```python
from build123d import *
from build123d.topology import SkipClean

# Parameters (mm, degrees)
SKETCH_1_R                   = 18
SKETCH_1_R_2                 = 1.3
SKETCH_1_R_3                 = 1.6
EXTRUDE_1_DEPTH              = 8
SKETCH_5_R                   = 2.1
CUT_EXTRUDE_1_DEPTH          = 6.6
HOLE_WIZARD_M3_2_D           = 3.6
HOLE_WIZARD_M3_2_CSINK_D     = 6.3
HOLE_WIZARD_M3_2_CSINK_ANGLE = 90
EXTRUDE_START                = 2
SKETCH_8_R                   = 10
SKETCH_8_R_2                 = 1.3
EXTRUDE_2_DEPTH              = 2
SKETCH_9_R                   = 10
SKETCH_9_R_2                 = 2.1
EXTRUDE_3_DEPTH              = 18
EXTRUDE_START_2              = -3.4
SKETCH_10_R                  = 2.1
SKETCH_10_R_2                = 1.25
EXTRUDE_4_DEPTH              = 3.4
SKETCH_11_R                  = 2.1
CUT_EXTRUDE_2_DEPTH          = 3.4


with BuildPart() as part:
    # 스케치1 → 보스-돌출1 (new body)
    with BuildSketch(Plane.XY):
        Circle(SKETCH_1_R)
        with Locations((0, 5.95)):
            Circle(SKETCH_1_R_2, mode=Mode.SUBTRACT)
        with Locations((5.95, 0)):
            Circle(SKETCH_1_R_2, mode=Mode.SUBTRACT)
        with Locations((0, -5.95)):
            Circle(SKETCH_1_R_2, mode=Mode.SUBTRACT)
        with Locations((-5.95, 0)):
            Circle(SKETCH_1_R_2, mode=Mode.SUBTRACT)
        with Locations((-13.249665953, 4.822484021)):
            Circle(SKETCH_1_R_3, mode=Mode.SUBTRACT)
        with Locations(Location((-13.249665953, -4.822484021, 0), (0, 0, 180))):
            Circle(SKETCH_1_R_3, mode=Mode.SUBTRACT)
        with Locations((10.801226648, 9.063305297)):
            Circle(SKETCH_1_R_3, mode=Mode.SUBTRACT)
        with Locations(Location((2.448439305, 13.885789317, 0), (0, 0, 180))):
            Circle(SKETCH_1_R_3, mode=Mode.SUBTRACT)
        with Locations((2.448439305, -13.885789317)):
            Circle(SKETCH_1_R_3, mode=Mode.SUBTRACT)
        with Locations(Location((10.801226648, -9.063305297, 0), (0, 0, 180))):
            Circle(SKETCH_1_R_3, mode=Mode.SUBTRACT)
    extrude(amount=EXTRUDE_1_DEPTH)

    # 스케치5 → 컷-돌출1 (cut)
    with BuildSketch(Plane.XY.offset(8)):
        with Locations((0, 5.95)):
            Circle(SKETCH_5_R)
        with Locations((0, -5.95)):
            Circle(SKETCH_5_R)
        with Locations((5.95, 0)):
            Circle(SKETCH_5_R)
        with Locations((-5.95, 0)):
            Circle(SKETCH_5_R)
    extrude(amount=-CUT_EXTRUDE_1_DEPTH, mode=Mode.SUBTRACT)

    # M3 접시 머리 나사용 카운터싱크2 (through all)
    with Locations(Plane(origin=(0, 0, 0), x_dir=(-1, 0, 0), z_dir=(0, 0, -1))):
        with Locations((-2.448439305, 13.885789317), (13.249665953, 4.822484021), (13.249665953, -4.822484021), (-2.448439305, -13.885789317), (-10.801226648, -9.063305297), (-10.801226648, 9.063305297)):
            CounterSinkHole(HOLE_WIZARD_M3_2_D / 2, HOLE_WIZARD_M3_2_CSINK_D / 2, counter_sink_angle=HOLE_WIZARD_M3_2_CSINK_ANGLE)

    # 스케치8 → 보스-돌출2 (add)
    with BuildSketch(Plane(origin=(0, 0, 0), x_dir=(-1, 0, 0), z_dir=(0, 0, -1)).offset(EXTRUDE_START)):
        with Locations(Location((0, 0, 0), (0, 0, 180))):
            Circle(SKETCH_8_R)
        with Locations((0, 5.95)):
            Circle(SKETCH_8_R_2, mode=Mode.SUBTRACT)
        with Locations((5.95, 0)):
            Circle(SKETCH_8_R_2, mode=Mode.SUBTRACT)
        with Locations((0, -5.95)):
            Circle(SKETCH_8_R_2, mode=Mode.SUBTRACT)
        with Locations((-5.95, 0)):
            Circle(SKETCH_8_R_2, mode=Mode.SUBTRACT)
    extrude(amount=-EXTRUDE_2_DEPTH)

    # 스케치9 → 보스-돌출3 (add)
    with SkipClean():  # the faces are left unmerged after this step: merging them gives an invalid solid
        with BuildSketch(Plane(origin=(0, 0, -2), x_dir=(-1, 0, 0), z_dir=(0, 0, -1))):
            with Locations(Location((0, 0, 0), (0, 0, 180))):
                Circle(SKETCH_9_R)
            with Locations(Location((5.95, 0, 0), (0, 0, 180))):
                Circle(SKETCH_9_R_2, mode=Mode.SUBTRACT)
            with Locations(Location((0, 5.95, 0), (0, 0, 180))):
                Circle(SKETCH_9_R_2, mode=Mode.SUBTRACT)
            with Locations(Location((-5.95, 0, 0), (0, 0, 180))):
                Circle(SKETCH_9_R_2, mode=Mode.SUBTRACT)
            with Locations(Location((0, -5.95, 0), (0, 0, 180))):
                Circle(SKETCH_9_R_2, mode=Mode.SUBTRACT)
        extrude(amount=EXTRUDE_3_DEPTH)

    # 스케치10 → 보스-돌출4 (add)
    # profile 1 of 4: a face of its own
    with SkipClean():  # the faces are left unmerged after this step: merging them gives an invalid solid
        with BuildSketch(Plane(origin=(0, 0, -20), x_dir=(-1, 0, 0), z_dir=(0, 0, -1)).offset(EXTRUDE_START_2)):
            with Locations((5.95, 0)):
                Circle(SKETCH_10_R)
            with Locations((5.95, 0)):
                Circle(SKETCH_10_R_2, mode=Mode.SUBTRACT)
        # profile 2 of 4: a face of its own
        with BuildSketch(Plane(origin=(0, 0, -20), x_dir=(-1, 0, 0), z_dir=(0, 0, -1)).offset(EXTRUDE_START_2)):
            with Locations((0, -5.95)):
                Circle(SKETCH_10_R)
            with Locations((0, -5.95)):
                Circle(SKETCH_10_R_2, mode=Mode.SUBTRACT)
        # profile 3 of 4: a face of its own
        with BuildSketch(Plane(origin=(0, 0, -20), x_dir=(-1, 0, 0), z_dir=(0, 0, -1)).offset(EXTRUDE_START_2)):
            with Locations((-5.95, 0)):
                Circle(SKETCH_10_R)
            with Locations((-5.95, 0)):
                Circle(SKETCH_10_R_2, mode=Mode.SUBTRACT)
        # profile 4 of 4: a face of its own
        with BuildSketch(Plane(origin=(0, 0, -20), x_dir=(-1, 0, 0), z_dir=(0, 0, -1)).offset(EXTRUDE_START_2)):
            with Locations((0, 5.95)):
                Circle(SKETCH_10_R)
            with Locations((0, 5.95)):
                Circle(SKETCH_10_R_2, mode=Mode.SUBTRACT)
        extrude(amount=EXTRUDE_4_DEPTH)

    # 스케치11 → 컷-돌출2 (cut)
    with BuildSketch(Plane.XY.offset(1.4)):
        with Locations((5.95, 0)):
            Circle(SKETCH_11_R)
        with Locations((0, -5.95)):
            Circle(SKETCH_11_R)
        with Locations((0, 5.95)):
            Circle(SKETCH_11_R)
        with Locations((-5.95, 0)):
            Circle(SKETCH_11_R)
    extrude(amount=-CUT_EXTRUDE_2_DEPTH, mode=Mode.SUBTRACT)


solid = part.part
```
Build history of the part. All positions in model axes, mm. A direction names the side the tool comes from. Coordinates: 2 decimals unless noted, no trailing zeros. Order: outer loops, then holes, each group sorted by start corner. A loop starts at its lowest first (then second) coordinate and runs counter-clockwise, first axis right, second up. Notation, with made-up numbers: (57.25, -32) -> (84.25, -32) arc R24 ccw to (84.25, -17) -> close; hole circle Ø3 at (37.25, 80). An arc over 180 degrees is marked (long way). Answer in a Markdown table with one row per item. Add a question column.
Q1. Band-saw the part on D-D, the plane z = -4.5. List the corners of the cut face in (x, y).
Q2. Band-saw the part on C-C, the plane x = -5.95. List the corners of the cut face in (y, z), then the cut area to 3 significant figures.
Q3. Wall check: line 1 along Y through (x, z) = (0, -10.75); line 2 along Y through (x, z) = (0, -18.9); line 3 along Z through (x, y) = (16, 0). Give the ranges that are in metal, low to high. Write a range as [from, to].
Q4. Band-saw the part on A-A, the plane y = 0. List the corners of the cut face in (x, z).
Q5. Drop flat-ended pins along their axis: pin 1 (1 mm diameter, centred on y = -8, z = -2, fed in from +X); pin 2 (1 mm diameter, centred on x = 0, y = -6.5, fed in from +Z); pin 3 (2 mm diameter, centred on x = 5.5, y = -0.5, fed in from +Z); pin 4 (12 mm diameter, centred on x = 11.5, z = -6.5, fed in from +Y). Give the stop position or say it passes through.
Q6. Band-saw the part on B-B, the plane z = 5.5. Give the number of separate pieces and of enclosed holes in the cut face, then the cut area to 3 significant figures.
Q7. Mould opens along X. For faces 1 (the face through (-2.343, 17.847, 3.944)), 2 (the face through (-1, -7, -16.6)), 3 (the face through (0, 0, -20)) say: +X half, -X half, draft (parallel to the pull), parting line (faces both ways), or undercut.
Q8. Which spindle directions (+Z, -Z, +X, -X, +Y, -Y) get a long thin tool onto all of the face, cutting with end or side? Do faces 4 (the face through (-11.6, 4.1, 4.7)), 5 (the face through (-7, -1, -16.6)). Say none if no direction does.
Answers follow:
| question | item | result |
|---|---|---|
| 1 | outline | circle Ø20 at (0, 0); hole circle Ø4.2 at (-5.95, 0); hole circle Ø4.2 at (0, -5.95); hole circle Ø4.2 at (0, 5.95); hole circle Ø4.2 at (5.95, 0) |
| 2 | outline | (-16.99, 0) -> (-8.04, 0) -> (-8.04, -20) -> (-1.25, -20) -> (-1.25, -16.6) -> (-2.1, -16.6) -> (-2.1, 8) -> (-16.99, 8) -> close; (1.25, -20) -> (8.04, -20) -> (8.04, 0) -> (16.99, 0) -> (16.99, 8) -> (2.1, 8) -> (2.1, -16.6) -> (1.25, -16.6) -> close |
| 2 | area | 481 mm^2 |
| 3 | line 1 | [-10, -8.05], [-3.85, 3.85], [8.05, 10] |
| 3 | line 2 | [-10, -7.2], [-4.7, 4.7], [7.2, 10] |
| 3 | line 3 | [0, 8] |
| 4 | outline | (-18, 0) -> (-10, 0) -> (-10, -20) -> (-7.2, -20) -> (-7.2, -16.6) -> (-8.05, -16.6) -> (-8.05, 8) -> (-18, 8) -> close; (-4.7, -20) -> (4.7, -20) -> (4.7, -16.6) -> (3.85, -16.6) -> (3.85, 8) -> (-3.85, 8) -> (-3.85, -16.6) -> (-4.7, -16.6) -> close; (7.2, -20) -> (10, -20) -> (10, 0) -> (18, 0) -> (18, 8) -> (8.05, 8) -> (8.05, -16.6) -> (7.2, -16.6) -> close |
| 5 | pin 1 | x = 6.61 |
| 5 | pin 2 | through |
| 5 | pin 3 | z = -16.6 |
| 5 | pin 4 | y = 8.35 |
| 6 | separate pieces | 1 |
| 6 | enclosed holes | 10 |
| 6 | area | 901 mm^2 |
| 7 | face 1 | parting line |
| 7 | face 2 | undercut |
| 7 | face 3 | draft |
| 8 | face 4 | +Z, -Z |
| 8 | face 5 | +Z |
